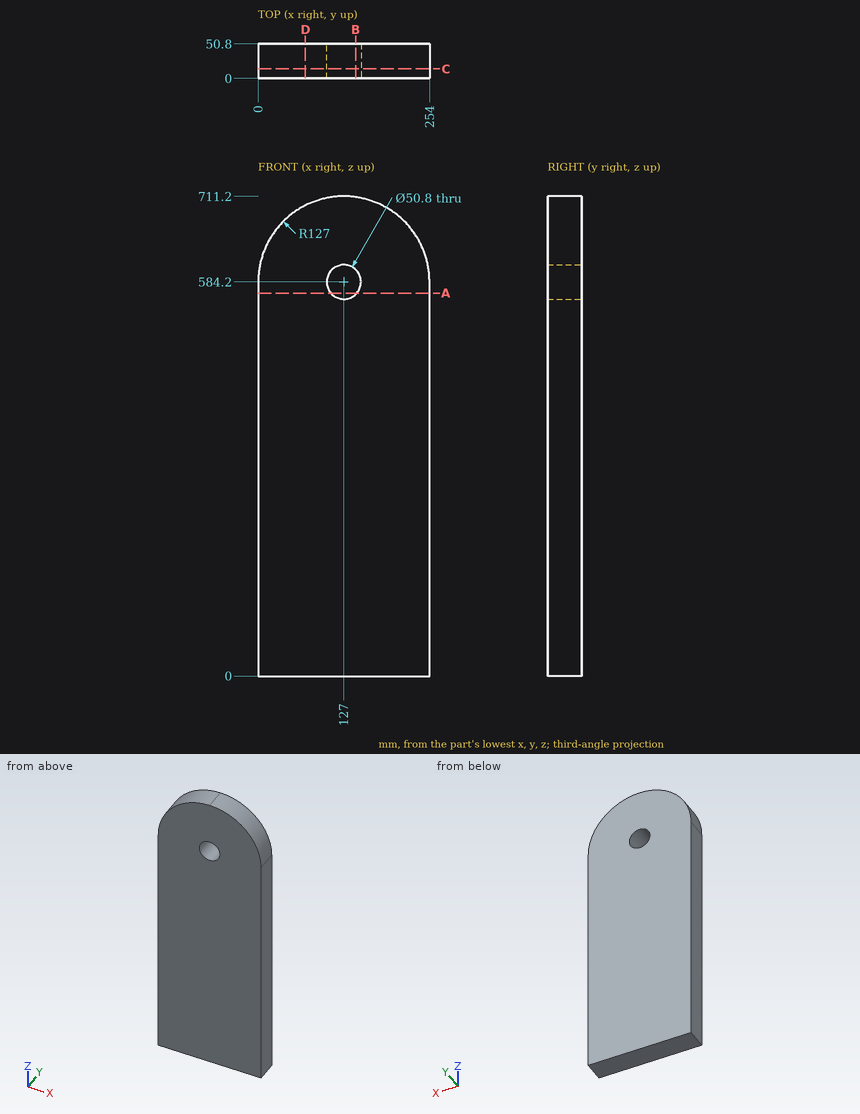
Part print with two shaded views. Sizes in mm from the minimum x, y, z corner. Round coordinates to 2 decimals unless told otherwise and drop trailing zeros. Order: outer loops, then holes, each group sorted by start corner. A loop starts at its lowest first (then second) coordinate and runs counter-clockwise, first axis right, second up. Notation, with made-up numbers: (50, 27.5) - (55, 27.5) arc R19 cw to (55, 51.5) - close; hole circle Ø5 at (33.25, -17.75). An arc over 180 degrees is marked (long way). Return JSON: item names as keys, results as strings.
(1) Pin check, flat tip, straight feed: pin 1 Ø4 at (x, y) = (209, 19.5) entering from -Z. Stop position of the tip, or through.
Answer key:
{"pin 1": "stops at z = 0"}
(2) Wall check: probe 1 along Z at (x, y) = (127, 11); probe 2 along X at (y, z) = (3, 583.5); probe 3 along X at (y, z) = (45, 602). Give the ranges that are in metal, low to high. Write a range as from..to.
Answer key:
{"probe 1": "z = 0..558.8, 609.6..711.2", "probe 2": "x = 0..101.61, 152.39..254", "probe 3": "x = 1.25..108.88, 145.12..252.75"}
(3) Cut at C-C (y = 14). Give the cut face in (x, z).
Answer key:
{"outline": "(0, 0) - (254, 0) - (254, 584.2) arc R127 ccw to (127, 711.2) arc R127 ccw to (0, 584.2) - close; hole circle Ø50.8 at (127, 584.2)"}
(4) Cut at D-D (x = 70). Give the cut face in (y, z), then the cut area to 3 significant figures.
Answer key:
{"outline": "(0, 0) - (50.8, 0) - (50.8, 697.69) - (0, 697.69) - close", "area": "35,400 mm^2"}
(5) Cut at B-B (x = 144.5). Give the cut face in (y, z).
Answer key:
{"outline": "(0, 0) - (50.8, 0) - (50.8, 565.79) - (0, 565.79) - close; (0, 602.61) - (50.8, 602.61) - (50.8, 709.99) - (0, 709.99) - close"}
(6) Cut at A-A (z = 567.5). Give the cut face in (x, y).
Answer key:
{"outline": "(0, 0) - (107.86, 0) - (107.86, 50.8) - (0, 50.8) - close; (146.14, 0) - (254, 0) - (254, 50.8) - (146.14, 50.8) - close"}
